```python
from build123d import *

# Parameters (mm, degrees)
F2_R     = 1.5
F3_DEPTH = 25


with BuildPart() as f1:
    # F0 (on Front) → F1 (revolve)
    with BuildSketch(Plane.XZ):
        with BuildLine():
            Line((1.5, 8), (1.5, 0))
            Line((1.5, 0), (2.95, 0))
            Line((2.95, 0), (2.95, 22.05))
            ThreePointArc((2.95, 22.05), (2.085965, 24.135965), (0, 25))
            Line((0, 25), (0, 8))
            Line((0, 8), (1.5, 8))
        make_face()
    revolve(axis=Axis((0, 0, 16.5), (0, 0, 1)))

    # F2 (on Front) → F3 (cut)
    with BuildSketch(Plane.XZ):
        with Locations((0, 13.5)):
            Circle(F2_R)
    extrude(amount=-F3_DEPTH, mode=Mode.SUBTRACT)


solid = f1.part
```
Work out the finished part from the listing and answer in its coordinate system (mm). A direction names the side the tool comes from. Give positions to 0.01 mm unless a question says otherwise; leave off trailing zeros. Loops run counter-clockwise (first coordinate to the right, second up) from the corner with the lowest first, then second, coordinate; pieces in that order, holes last. Notation, with made-up numbers: (4.25, -4.75) -> (26.25, -4.75) arc R21 cw to (26.25, 34.25) -> close; hole circle Ø4 at (6, 36.5). An arc over 180 degrees is marked (long way). One line per question, with ' | ' between items. Start each with the question number.
1) Section A-A, the plane x = 0 is taken. Determine the outline of the cut face in (y, z), then the cut area to 3 significant figures.
2) Section C-C, the plane z = 11.5 is taken. Determine the outline of the cut face in (x, y), then the cut area to 3 significant figures.
3) Each of these flat-tipped pins is pushed along its axis until it touches: pin 1 (0.9 mm diameter, centred on x = -0.5, y = 0, fed in from -Z); pin 2 (2 mm diameter, centred on y = -1.5, z = 16.5, fed in from -X); pin 3 (1 mm diameter, centred on x = 1.5, z = 22, fed in from -Y). Where does it stop, or does it pass through?
4) For faces 4 (the face through (0, 0, 8)), 5 (the face through (1.386, 1.454, 12.925)), determine the directions among +Z, -Z, +X, -X, +Y, -Y from which every point of the face is accessible in a straight line to the end or side of a thin tool.
5) Straight lines are drawn through the part: L1, parallel to Y at x = 0, z = 5; L2, parallel to Z at x = -1.15, y = 2.4; L3, parallel to Z at x = -1.35, y = 1.85. For each, find the intervals that lie inside material, in ascending order.
6) Section B-B, the plane y = -0.5 is taken. Determine the outline of the cut face in (x, z), then the cut area to 3 significant figures.
7) Section D-D, the plane x = 1.85 is taken. Determine the outline of the cut face in (y, z), then the cut area to 3 significant figures.
8) Determine the mould class of faces 1 (the face through (-1.3, -1.3, 0)), 2 (the face through (0, 0, 14)), 3 (the face through (-0.64, -2.88, 11.18)) for opening direction X: +X half, -X half, draft (parallel to the pull), parting line (faces both ways), or undercut.
Resolved:
1) outline: (-2.95, 0) -> (-1.5, 0) -> (-1.5, 8) -> (1.5, 8) -> (1.5, 0) -> (2.95, 0) -> (2.95, 12) -> (0, 12) -> (0, 15) -> (2.95, 15) -> (2.95, 22.05) arc R2.95 ccw to (-2.95, 22.05) -> close | area: 111 mm2
2) outline: circle Ø5.9 at (0, 0) | area: 27.3 mm2
3) pin 1: z = 8 | pin 2: x = -2.91 | pin 3: y = -2.78
4) face 4: -Z | face 5: +Y
5) L1: -2.95 to -1.5, 1.5 to 2.95 | L2: 0 to 12.54, 14.46 to 23.32 | L3: 0 to 12.85, 14.15 to 23.91
6) outline: (-2.91, 0) -> (-1.41, 0) -> (-1.41, 8) -> (1.41, 8) -> (1.41, 0) -> (2.91, 0) -> (2.91, 22.05) arc R2.91 ccw to (-2.91, 22.05) -> close | area: 119 mm2
7) outline: (-2.3, 0) -> (2.3, 0) -> (2.3, 22.05) arc R2.3 ccw to (-2.3, 22.05) -> close | area: 110 mm2
8) face 1: draft | face 2: undercut | face 3: parting line
